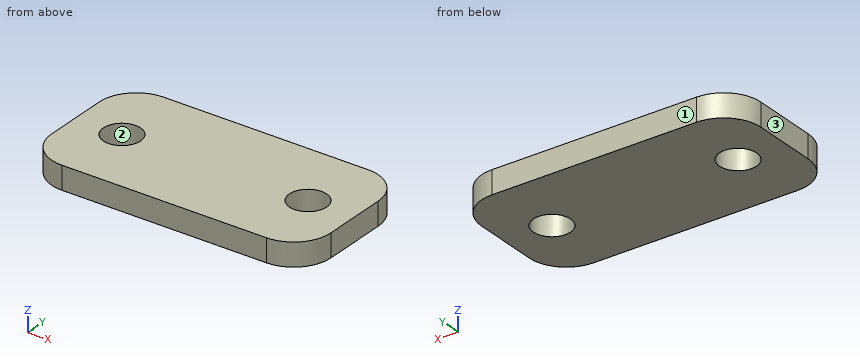
from build123d import *

# Parameters (mm, degrees)
SKETCH1_R           = 4
BOSS_EXTRUDE1_DEPTH = 5


with BuildPart() as part:
    # Sketch1 → Boss-Extrude1 (new body)
    with BuildSketch(Plane.XY):
        with BuildLine():
            Line((22, -15), (-22, -15))
            ThreePointArc((-22, -15), (-27.656854249, -12.656854249), (-30, -7))
            Line((-30, -7), (-30, 7))
            ThreePointArc((-30, 7), (-27.656854249, 12.656854249), (-22, 15))
            Line((-22, 15), (22, 15))
            ThreePointArc((22, 15), (27.656854249, 12.656854249), (30, 7))
            Line((30, 7), (30, -7))
            ThreePointArc((30, -7), (27.656854249, -12.656854249), (22, -15))
        make_face()
        with Locations((-20, 0)):
            Circle(SKETCH1_R, mode=Mode.SUBTRACT)
        with Locations(Location((20, 0, 0), (0, 0, 180))):
            Circle(SKETCH1_R, mode=Mode.SUBTRACT)
    extrude(amount=BOSS_EXTRUDE1_DEPTH)


solid = part.part
The model under review builds one solid part; all positions refer to its coordinate system, in mm. Face numbers are marked on the shaded views. Round coordinates to 2 decimals unless told otherwise and drop trailing zeros. Write each loop counter-clockwise with the first axis right and the second up, starting at its lowest first coordinate (ties: lowest second). Pieces come first, ordered by that corner, then holes. Notation, with made-up numbers: M 89.25,60 L 129.25,60 A11 cw 129.25,73 Z; hole C 62.25,51.5 d5. An arc over 180 degrees is marked long. Answer as CSV lines item,"result". Start each with the question number.
Q1. Consider section B-B, the plane z = 0.6. Give the boundary of the cut face in (x, y).
Q2. The part is to be moulded in two halves that separate along X. For the marked faces 1, 2 and 3, say which applies: +X half, -X half, draft (parallel to the pull), parting line (faces both ways), or undercut.
Q3. Consider section D-D, the plane y = -10.25. Give the boundary of the cut face in (x, z).
Q4. Consider section C-C, the plane y = 0. Give the boundary of the cut face in (x, z), then the cut area to 3 significant figures.
Q5. Wall thickness on line 1 along Y through (x, z) = (20, 2.65); line 2 along X through (y, z) = (-1.25, 4.2); line 3 along X through (y, z) = (1, 3.5): over which ranges is each line inside the solid? List them lowest first.
Q6. Consider section A-A, the plane x = 20. Give the boundary of the cut face in (y, z).
Result set:
1,outline,"M -30,-7 A8 ccw -22,-15 L 22,-15 A8 ccw 30,-7 L 30,7 A8 ccw 22,15 L -22,15 A8 ccw -30,7 Z; hole C -20,0 d8; hole C 20,0 d8"
2,face 1,"draft"
2,face 2,"undercut"
2,face 3,"-X half"
3,outline,"M -29.31,0 L 29.31,0 L 29.31,5 L -29.31,5 Z"
4,outline,"M -30,0 L -24,0 L -24,5 L -30,5 Z; M -16,0 L 16,0 L 16,5 L -16,5 Z; M 24,0 L 30,0 L 30,5 L 24,5 Z"
4,area,"220 mm²"
5,line 1,"y = -15 to -4, 4 to 15"
5,line 2,"x = -30 to -23.8, -16.2 to 16.2, 23.8 to 30"
5,line 3,"x = -30 to -23.87, -16.13 to 16.13, 23.87 to 30"
6,outline,"M -15,0 L -4,0 L -4,5 L -15,5 Z; M 4,0 L 15,0 L 15,5 L 4,5 Z"
